Check sheet for the drawn part. Datum: minimum x, y, z corner. Units: mm. A direction names the side the tool comes from. Round coordinates to 2 decimals unless told otherwise and drop trailing zeros. Write each loop counter-clockwise with the first axis right and the second up, starting at its lowest first coordinate (ties: lowest second). Pieces come first, ordered by that corner, then holes. Notation, with made-up numbers: (28.5, 63.5) -> (73.5, 63.5) arc R21 cw to (73.5, 85.5) -> close; hole circle Ø3 at (-14, 64.5). An arc over 180 degrees is marked (long way). Use a Markdown table: item, result.
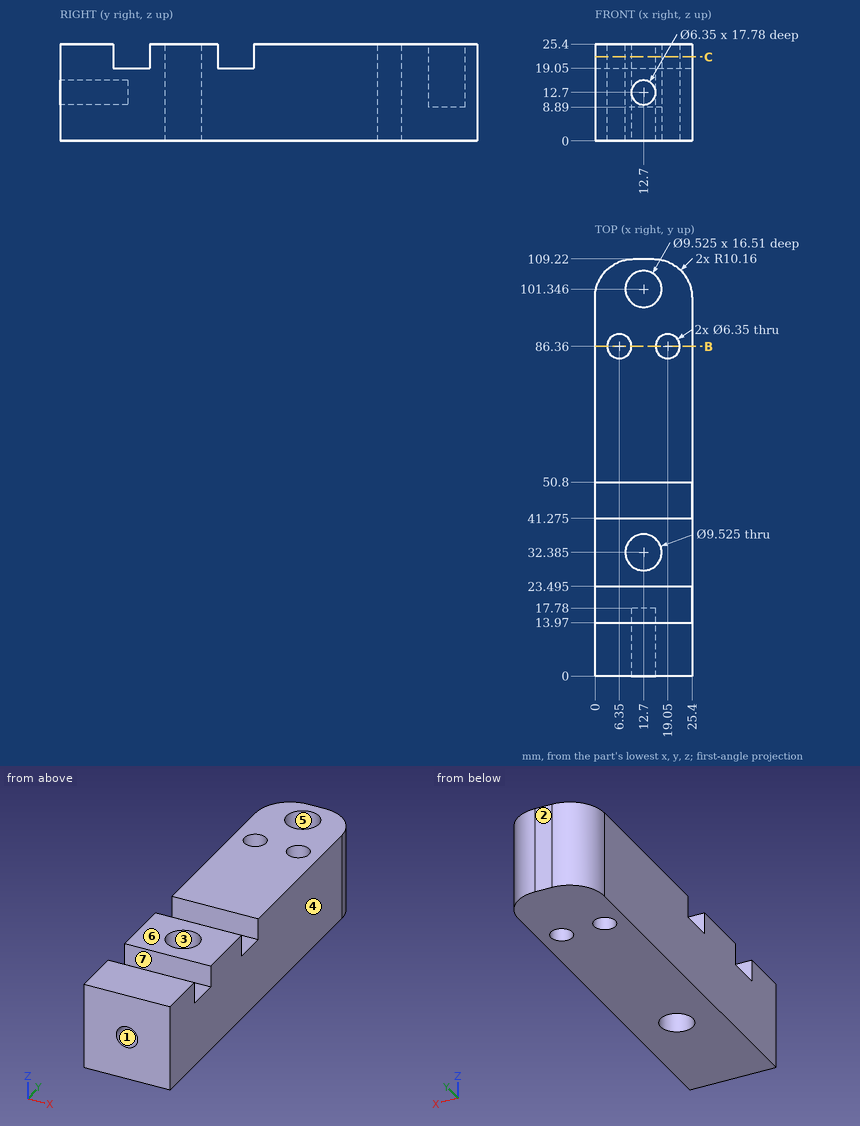
(1) Thickness scan on line 1 (Y direction, x = 12.7, z = 9.25); line 2 (Y direction, x = 12.7, z = 19.5) (1 decimal); line 3 (X direction, y = 88, z = 6.75). Record the ranges inside material, lowest first.
A:
| item | result |
|---|---|
| line 1 | y = 0 to 27.62, 37.15 to 96.58, 106.11 to 109.22 |
| line 2 | y = 0 to 14, 23.5 to 27.6, 37.1 to 41.3, 50.8 to 96.6, 106.1 to 109.2 |
| line 3 | x = 0 to 3.63, 9.07 to 16.33, 21.77 to 25.4 |
(2) Gauge pin test, flat ends, axial feed: pin 1 Ø5 at (x, y) = (8.5, 45.5) entering from +Z; pin 2 Ø3 at (x, y) = (12, 100) entering from +Z; pin 3 Ø5 at (x, y) = (19.05, 86.36) entering from -Z. Record the tip position at first contact, or that the pin passes through.
A:
| item | result |
|---|---|
| pin 1 | stops at z = 19.05 |
| pin 2 | stops at z = 8.89 |
| pin 3 | passes through |
(3) Section check B-B on y = 86.36. Record the cut outline in (x, z) (3 decimals), plus the area to 3 significant figures.
A:
| item | result |
|---|---|
| outline | (0, 0) -> (3.175, 0) -> (3.175, 25.4) -> (0, 25.4) -> close; (9.525, 0) -> (15.875, 0) -> (15.875, 25.4) -> (9.525, 25.4) -> close; (22.225, 0) -> (25.4, 0) -> (25.4, 25.4) -> (22.225, 25.4) -> close |
| area | 323 mm2 |
(4) Release check for a two-part mould opening along X. For the marked faces 1, 2, 3 and 4 record: +X half, -X half, draft (parallel to the pull), parting line (faces both ways), or undercut.
A:
| item | result |
|---|---|
| face 1 | undercut |
| face 2 | draft |
| face 3 | undercut |
| face 4 | +X half |
(5) Section check C-C on z = 22. State how many separate pieces and enclosed holes the cut face has, plus the area to 3 significant figures.
A:
| item | result |
|---|---|
| separate pieces | 3 |
| enclosed holes | 4 |
| area | 2,040 mm2 |
(6) Access from +Z, -Z, +X, -X, +Y, -Y to the whole of each face (thin tool, end or side, straight path). Record for the marked faces 5, 6 and 7.
A:
| item | result |
|---|---|
| face 5 | +Z |
| face 6 | +Z, +X, -X, +Y, -Y |
| face 7 | +Z, +X, -X |
